from build123d import *

# Parameters (mm, degrees)
SKETCH_1_W          = 250
SKETCH_1_H          = 50
EXTRUDE_1_DEPTH     = 3
CUT_EXTRUDE_1_REACH = 129.511
SKETCH_3_R          = 1.6
FILLET_1_R          = 2


with BuildPart() as part:
    # 草图1 → 凸台-拉伸1 (new body)
    with BuildSketch(Plane(origin=(0, 0, 0), x_dir=(1, 0, 0), z_dir=(0, 1, 0))):
        Rectangle(SKETCH_1_W, SKETCH_1_H)
    extrude(amount=EXTRUDE_1_DEPTH)

    # 草图3 → 切除-拉伸1 (cut, up to next)
    with BuildSketch(Plane(origin=(0, 3, 0), x_dir=(1, 0, 0), z_dir=(0, 1, 0)), mode=Mode.PRIVATE) as cut_extrude_1_sk1:
        with Locations(Location((-117.5, 10, 0), (0, 0, 270))):
            Circle(SKETCH_3_R)
    cut_extrude_1_tool1 = extrude(cut_extrude_1_sk1.sketch, amount=-CUT_EXTRUDE_1_REACH, mode=Mode.PRIVATE) & part.part
    # 草图3 → 切除-拉伸1 (cut, up to next)
    with BuildSketch(Plane(origin=(0, 3, 0), x_dir=(1, 0, 0), z_dir=(0, 1, 0)), mode=Mode.PRIVATE) as cut_extrude_1_sk2:
        with Locations(Location((-102.5, 10, 0), (0, 0, 270))):
            Circle(SKETCH_3_R)
    cut_extrude_1_tool2 = extrude(cut_extrude_1_sk2.sketch, amount=-CUT_EXTRUDE_1_REACH, mode=Mode.PRIVATE) & part.part
    # 草图3 → 切除-拉伸1 (cut, up to next)
    with BuildSketch(Plane(origin=(0, 3, 0), x_dir=(1, 0, 0), z_dir=(0, 1, 0)), mode=Mode.PRIVATE) as cut_extrude_1_sk3:
        with Locations(Location((-102.5, -10, 0), (0, 0, 270))):
            Circle(SKETCH_3_R)
    cut_extrude_1_tool3 = extrude(cut_extrude_1_sk3.sketch, amount=-CUT_EXTRUDE_1_REACH, mode=Mode.PRIVATE) & part.part
    # 草图3 → 切除-拉伸1 (cut, up to next)
    with BuildSketch(Plane(origin=(0, 3, 0), x_dir=(1, 0, 0), z_dir=(0, 1, 0)), mode=Mode.PRIVATE) as cut_extrude_1_sk4:
        with Locations(Location((-117.5, -10, 0), (0, 0, 270))):
            Circle(SKETCH_3_R)
    cut_extrude_1_tool4 = extrude(cut_extrude_1_sk4.sketch, amount=-CUT_EXTRUDE_1_REACH, mode=Mode.PRIVATE) & part.part
    # 草图3 → 切除-拉伸1 (cut, up to next)
    with BuildSketch(Plane(origin=(0, 3, 0), x_dir=(1, 0, 0), z_dir=(0, 1, 0)), mode=Mode.PRIVATE) as cut_extrude_1_sk5:
        with Locations(Location((117.5, -10, 0), (0, 0, 270))):
            Circle(SKETCH_3_R)
    cut_extrude_1_tool5 = extrude(cut_extrude_1_sk5.sketch, amount=-CUT_EXTRUDE_1_REACH, mode=Mode.PRIVATE) & part.part
    # 草图3 → 切除-拉伸1 (cut, up to next)
    with BuildSketch(Plane(origin=(0, 3, 0), x_dir=(1, 0, 0), z_dir=(0, 1, 0)), mode=Mode.PRIVATE) as cut_extrude_1_sk6:
        with Locations(Location((102.5, 10, 0), (0, 0, 270))):
            Circle(SKETCH_3_R)
    cut_extrude_1_tool6 = extrude(cut_extrude_1_sk6.sketch, amount=-CUT_EXTRUDE_1_REACH, mode=Mode.PRIVATE) & part.part
    # 草图3 → 切除-拉伸1 (cut, up to next)
    with BuildSketch(Plane(origin=(0, 3, 0), x_dir=(1, 0, 0), z_dir=(0, 1, 0)), mode=Mode.PRIVATE) as cut_extrude_1_sk7:
        with Locations(Location((117.5, 10, 0), (0, 0, 270))):
            Circle(SKETCH_3_R)
    cut_extrude_1_tool7 = extrude(cut_extrude_1_sk7.sketch, amount=-CUT_EXTRUDE_1_REACH, mode=Mode.PRIVATE) & part.part
    # 草图3 → 切除-拉伸1 (cut, up to next)
    with BuildSketch(Plane(origin=(0, 3, 0), x_dir=(1, 0, 0), z_dir=(0, 1, 0)), mode=Mode.PRIVATE) as cut_extrude_1_sk8:
        with Locations(Location((102.5, -10, 0), (0, 0, 270))):
            Circle(SKETCH_3_R)
    cut_extrude_1_tool8 = extrude(cut_extrude_1_sk8.sketch, amount=-CUT_EXTRUDE_1_REACH, mode=Mode.PRIVATE) & part.part
    add(cut_extrude_1_tool1.solids().sort_by_distance((-117.5, 3, -10))[0], mode=Mode.SUBTRACT)
    add(cut_extrude_1_tool2.solids().sort_by_distance((-102.5, 3, -10))[0], mode=Mode.SUBTRACT)
    add(cut_extrude_1_tool3.solids().sort_by_distance((-102.5, 3, 10))[0], mode=Mode.SUBTRACT)
    add(cut_extrude_1_tool4.solids().sort_by_distance((-117.5, 3, 10))[0], mode=Mode.SUBTRACT)
    add(cut_extrude_1_tool5.solids().sort_by_distance((117.5, 3, 10))[0], mode=Mode.SUBTRACT)
    add(cut_extrude_1_tool6.solids().sort_by_distance((102.5, 3, -10))[0], mode=Mode.SUBTRACT)
    add(cut_extrude_1_tool7.solids().sort_by_distance((117.5, 3, -10))[0], mode=Mode.SUBTRACT)
    add(cut_extrude_1_tool8.solids().sort_by_distance((102.5, 3, 10))[0], mode=Mode.SUBTRACT)

    # 圆角1
    fillet_1_edges = [part.edges().sort_by_distance(p)[0] for p in [
        (125, 1.5, 25),
        (-125, 1.5, 25),
        (-125, 1.5, -25),
        (125, 1.5, -25),
    ]]
    fillet(fillet_1_edges, radius=FILLET_1_R)


solid = part.part
Read the model definition and answer for the solid it produces. Units are mm, in the model's axes. Give positions to 0.01 mm unless a question says otherwise; leave off trailing zeros. Return JSON: item names as keys, results as strings.
Q1. For a pull along Y with two mould halves and no side action, classify faces 1 (the face through (-2, 3, 0)), 2 (the face through (-2, 0, 0)) as released by +Y, released by -Y, zero draft, split by the parting line, or undercut.
Reply:
{"face 1": "released by +Y", "face 2": "released by -Y"}
Q2. Given P1, Ø3, axis at x = -102.5, z = 10, coming from the -Y side, flat-ended and moving along its own axis, determine where the tip first touches the part or whether it passes through.
Reply:
{"P1": "through"}
Q3. Consider line 1 along Z through (x, y) = (-102.5, 2.3); line 2 along X through (y, z) = (1.8, 10); line 3 along X through (y, z) = (0.6, 10.5). Determine where each line is inside the solid, lowest interval first. Write a range as [from, to].
Reply:
{"line 1": "[-25, -11.6], [-8.4, 8.4], [11.6, 25]", "line 2": "[-125, -119.1], [-115.9, -104.1], [-100.9, 100.9], [104.1, 115.9], [119.1, 125]", "line 3": "[-125, -119.02], [-115.98, -104.02], [-100.98, 100.98], [104.02, 115.98], [119.02, 125]"}
